```python
from build123d import *

# Parameters (mm, degrees)
SKETCH2_W           = 50.8
SKETCH2_H           = 105.799998966
SKETCH2_R           = 9.5885
SKETCH2_R_2         = 14.2875
SKETCH2_R_3         = 2.38125
BOSS_EXTRUDE1_DEPTH = 6.35
SKETCH6_R           = 2.0828
CUT_EXTRUDE1_DEPTH  = 51.8


with BuildPart() as part:
    # Sketch2 → Boss-Extrude1 (new body)
    with BuildSketch(Plane.XY):
        with Locations((0, -27.499999483)):
            Rectangle(SKETCH2_W, SKETCH2_H)
        Circle(SKETCH2_R, mode=Mode.SUBTRACT)
        with Locations((0, -54.999998966)):
            Circle(SKETCH2_R_2, mode=Mode.SUBTRACT)
        with Locations((-17.960512242, -17.960512242)):
            Circle(SKETCH2_R_3, mode=Mode.SUBTRACT)
        with Locations((17.960512242, 17.960512242)):
            Circle(SKETCH2_R_3, mode=Mode.SUBTRACT)
    extrude(amount=BOSS_EXTRUDE1_DEPTH)

    # Sketch6 → Cut-Extrude1 (cut, through all)
    with BuildSketch(Plane(origin=(25.4, 0, 0), x_dir=(0, 0, -1), z_dir=(1, 0, 0))):
        with Locations((-3.175, -65.159998966)):
            Circle(SKETCH6_R)
        with Locations((-3.175, -46.109998966)):
            Circle(SKETCH6_R)
    extrude(amount=-CUT_EXTRUDE1_DEPTH, mode=Mode.SUBTRACT)


solid = part.part
```
Design review of the part built by this model. Coordinates are the model's own, in mm. Give positions to 0.01 mm unless a question says otherwise; leave off trailing zeros. Write each loop counter-clockwise with the first axis right and the second up, starting at its lowest first coordinate (ties: lowest second). Pieces come first, ordered by that corner, then holes. Notation, with made-up numbers: (53.25, 32.5) - (66.25, 32.5) arc R24 ccw to (66.25, 57.5) - close; hole circle Ø5 at (64, 18). An arc over 180 degrees is marked (long way). Return JSON: item names as keys, results as strings. Group by question number.
(1) We need section D-D, the plane y = -43. Give the boundary of the cut face in (x, z), then the cut area to 3 significant figures.
(2) We need section C-C, the plane y = 0. Give the boundary of the cut face in (x, z), then the cut area to 3 significant figures.
(3) We need section A-A, the plane z = 3.5. Give the boundary of the cut face in (x, y) (1 decimal), then the cut area to 3 significant figures.
(4) Mouldability with a two-part tool opening along Y and no side actions: class faces 1 (the flat face through (0, 25.4, 3)), 2 (the cylindrical face through (18.5, -67.2, 3.6)), 3 (the flat face through (0, -27, 0)) as +Y half, -Y half, draft (parallel to the pull), parting line (faces both ways), or undercut.
(5) We need section B-B, the plane x = 0. Give the boundary of the cut face in (y, z).
(6) Insertion check: pin 1 (2 mm diameter, centred on x = 20.5, y = 7.5, fed in from -Z). The pin has a flat end and moves straight along its axis. Give the tip position at first contact, or say it passes through.
(7) To check wall thickness, follow probe 1 along Y at (x, z) = (-2.5, 1.5); probe 2 along Y at (x, z) = (14.5, 1.5); probe 3 along Y at (x, z) = (-17.5, 2). State the ranges of each line that lie inside material, in increasing order.
Reported:
{
 "1": {"outline": "(-25.4, 0) - (-7.75, 0) - (-7.75, 6.35) - (-25.4, 6.35) - close; (7.75, 0) - (25.4, 0) - (25.4, 6.35) - (7.75, 6.35) - close", "area": "224 mm2"},
 "2": {"outline": "(-25.4, 0) - (-9.59, 0) - (-9.59, 6.35) - (-25.4, 6.35) - close; (9.59, 0) - (25.4, 0) - (25.4, 6.35) - (9.59, 6.35) - close", "area": "201 mm2"},
 "3": {"outline": "(-25.4, -80.4) - (25.4, -80.4) - (25.4, -67.2) - (7.4, -67.2) arc R14.3 cw to (-7.4, -67.2) - (-25.4, -67.2) - close; (-25.4, -63.1) - (-11.8, -63.1) arc R14.3 cw to (-12.5, -48.2) - (-25.4, -48.2) - close; (-25.4, -44.1) - (-9.2, -44.1) arc R14.3 cw to (9.2, -44.1) - (25.4, -44.1) - (25.4, 25.4) - (-25.4, 25.4) - close; (11.8, -63.1) - (25.4, -63.1) - (25.4, -48.2) - (12.5, -48.2) arc R14.3 cw to start; hole circle Ø4.8 at (-18, -18); hole circle Ø19.2 at (0, 0); hole circle Ø4.8 at (18, 18)", "area": "4,160 mm2"},
 "4": {"face 1": "+Y half", "face 2": "undercut", "face 3": "draft"},
 "5": {"outline": "(-80.4, 0) - (-69.29, 0) - (-69.29, 6.35) - (-80.4, 6.35) - close; (-40.71, 0) - (-9.59, 0) - (-9.59, 6.35) - (-40.71, 6.35) - close; (9.59, 0) - (25.4, 0) - (25.4, 6.35) - (9.59, 6.35) - close"},
 "6": {"pin 1": "stops at z = 0"},
 "7": {"probe 1": "y = -80.4 to -69.07, -40.93 to -9.26, 9.26 to 25.4", "probe 2": "y = -80.4 to -66.4, -63.92 to -47.35, -44.87 to 25.4", "probe 3": "y = -80.4 to -66.88, -63.44 to -47.83, -44.39 to -20.3, -15.62 to 25.4"}
}
